The listing builds one solid part. Answer for the finished solid, in the listing's coordinates (mm). Face numbers are marked on the shaded views. A direction names the side the tool comes from. Give positions to 0.01 mm unless a question says otherwise; leave off trailing zeros. Write each loop counter-clockwise with the first axis right and the second up, starting at its lowest first coordinate (ties: lowest second). Pieces come first, ordered by that corner, then holes. Notation, with made-up numbers: M 29,66 L 53,66 A15 ccw 53,74 Z; hole C -6,29 d5. An arc over 180 degrees is marked long. Answer as a JSON object with one key per item and string values.
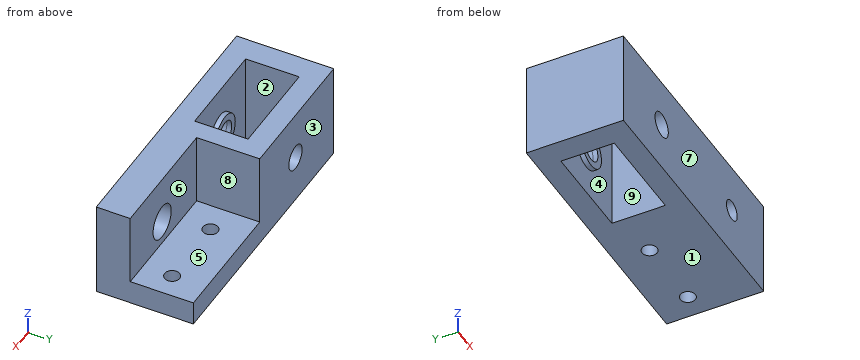
```python
from build123d import *

# Parameters (mm, degrees)
SKETCH_W        = 55
SKETCH_H        = 20
SKETCH_R        = 1.55
SKETCH_W_2      = 20
SKETCH_H_2      = 11
PAD_DEPTH       = 10
SKETCH001_R     = 2.6
POCKET_DEPTH    = 5
SKETCH002_R     = 2.6
POCKET001_DEPTH = 5
SKETCH003_R     = 4
SKETCH003_R_2   = 2.6
PAD001_DEPTH    = 1
SKETCH004_R     = 4
SKETCH004_R_2   = 2.6
PAD002_DEPTH    = 1
SKETCH005_W     = 26
SKETCH005_H     = 15
POCKET002_DEPTH = 13
SKETCH006_R     = 2.1
POCKET003_DEPTH = 7
SKETCH007_R     = 3.55
SKETCH007_R_2   = 2.1
POCKET004_DEPTH = 3


with BuildPart() as part:
    # Sketch → Pad (new body, symmetric)
    with BuildSketch(Plane.XY):
        Rectangle(SKETCH_W, SKETCH_H)
        with Locations((7.5, 3)):
            Circle(SKETCH_R, mode=Mode.SUBTRACT)
        with Locations((22.5, 3)):
            Circle(SKETCH_R, mode=Mode.SUBTRACT)
        with Locations((-12.5, 0)):
            Rectangle(SKETCH_W_2, SKETCH_H_2, mode=Mode.SUBTRACT)
    extrude(amount=PAD_DEPTH, both=True)

    # Sketch001 → Pocket (cut)
    with BuildSketch(Plane.XZ.offset(-5.5)):
        with Locations((-12.5, 0)):
            Circle(SKETCH001_R)
    extrude(amount=-POCKET_DEPTH, mode=Mode.SUBTRACT)

    # Sketch002 → Pocket001 (cut)
    with BuildSketch(Plane(origin=(0, -5.5, 0), x_dir=(-1, 0, 0), z_dir=(0, 1, 0))):
        with Locations((12.5, 0)):
            Circle(SKETCH002_R)
    extrude(amount=-POCKET001_DEPTH, mode=Mode.SUBTRACT)

    # Sketch003 → Pad001 (new body)
    with BuildSketch(Plane(origin=(0, -5.5, 0), x_dir=(-1, 0, 0), z_dir=(0, 1, 0))):
        with Locations((12.5, 0)):
            Circle(SKETCH003_R)
        with Locations((12.5, 0)):
            Circle(SKETCH003_R_2, mode=Mode.SUBTRACT)
    extrude(amount=PAD001_DEPTH)

    # Sketch004 → Pad002 (new body)
    with BuildSketch(Plane.XZ.offset(-5.5)):
        with Locations((-12.5, 0)):
            Circle(SKETCH004_R)
        with Locations((-12.5, 0)):
            Circle(SKETCH004_R_2, mode=Mode.SUBTRACT)
    extrude(amount=PAD002_DEPTH)

    # Sketch005 → Pocket002 (cut)
    with BuildSketch(Plane(origin=(0, 10, 0), x_dir=(-1, 0, 0), z_dir=(0, 1, 0))):
        with Locations((-14.5, 2.5)):
            Rectangle(SKETCH005_W, SKETCH005_H)
    extrude(amount=-POCKET002_DEPTH, mode=Mode.SUBTRACT)

    # Sketch006 → Pocket003 (cut)
    with BuildSketch(Plane(origin=(0, -3, 0), x_dir=(-1, 0, 0), z_dir=(0, 1, 0))):
        with Locations((-15, 0)):
            Circle(SKETCH006_R)
    extrude(amount=-POCKET003_DEPTH, mode=Mode.SUBTRACT)

    # Sketch007 → Pocket004 (cut)
    with BuildSketch(Plane(origin=(0, -3, 0), x_dir=(-1, 0, 0), z_dir=(0, 1, 0))):
        with Locations((-15, 0)):
            Circle(SKETCH007_R)
        with Locations((-15, 0)):
            Circle(SKETCH007_R_2, mode=Mode.SUBTRACT)
    extrude(amount=-POCKET004_DEPTH, mode=Mode.SUBTRACT)


solid = part.part
```
1. A cutting plane is placed at B-B, the plane x = 15. Give the vertices of the cut face in (y, z).
Verdict:
{"outline": "M -10,-10 L 10,-10 L 10,-5 L -3,-5 L -3,-3.55 L -6,-3.55 L -6,-2.1 L -10,-2.1 Z; M -10,2.1 L -6,2.1 L -6,3.55 L -3,3.55 L -3,10 L -10,10 Z"}
2. The mould has two halves that part along Y. Classify the marked faces 6, 7, 8 and 9: released by +Y, released by -Y, zero draft, split by the parting line, or undercut.
Verdict:
{"face 6": "released by +Y", "face 7": "released by -Y", "face 8": "zero draft", "face 9": "undercut"}
3. Flat-ended cylindrical pins translate along their axes: pin 1 (12 mm diameter, centred on x = 14, z = 3.5, fed in from +Y); pin 2 (12 mm diameter, centred on x = 10, y = 4, fed in from +Z); pin 3 (5.5 mm diameter, centred on y = 2.5, z = 4.5, fed in from +X). Find the tip coordinate at first contact, or state that the pin passes through.
Verdict:
{"pin 1": "stops at y = -3", "pin 2": "stops at z = -5", "pin 3": "stops at x = 1.5"}
4. Consider line 1 along X through (y, z) = (3, -8.25); line 2 along Z through (x, y) = (-12.5, -7.7); line 3 along Y through (x, z) = (-15, 8.75). Determine where each line is inside the solid, lowest interval first.
Verdict:
{"line 1": "x = -27.5 to -22.5, -2.5 to 5.95, 9.05 to 20.95, 24.05 to 27.5", "line 2": "z = -10 to -2.6, 2.6 to 10", "line 3": "y = -10 to -5.5, 5.5 to 10"}
5. A cutting plane is placed at D-D, the plane z = 0. Count the separate pieces of the cut face and the enclosed holes in it, plus the area to 3 significant figures.
Verdict:
{"separate pieces": "3", "enclosed holes": "0", "area": "463 mm2"}
6. A cutting plane is placed at C-C, the plane y = 3. Give the vertices of the cut face in (x, z), plus the area to 3 significant figures.
Verdict:
{"outline": "M -27.5,-10 L -22.5,-10 L -22.5,10 L -27.5,10 Z; M -2.5,-10 L 5.95,-10 L 5.95,-5 L 1.5,-5 L 1.5,10 L -2.5,10 Z; M 9.05,-10 L 20.95,-10 L 20.95,-5 L 9.05,-5 Z; M 24.05,-10 L 27.5,-10 L 27.5,-5 L 24.05,-5 Z", "area": "279 mm2"}
7. A cutting plane is placed at A-A, the plane y = 0.75. Give the vertices of the cut face in (x, z), plus the area to 3 significant figures.
Verdict:
{"outline": "M -27.5,-10 L -22.5,-10 L -22.5,10 L -27.5,10 Z; M -2.5,-10 L 27.5,-10 L 27.5,-5 L 1.5,-5 L 1.5,10 L -2.5,10 Z", "area": "310 mm2"}
8. For the marked faces 1, 2, 3, 4 and 5, determine the directions among +Z, -Z, +X, -X, +Y, -Y from which every point of the face is accessible in a straight line to the end or side of a thin tool.
Verdict:
{"face 1": "-Z, +X, -X, +Y, -Y", "face 2": "+Z, -Z", "face 3": "+Z, -Z, +X, -X, +Y", "face 4": "none", "face 5": "+Z, +X, +Y"}
